from build123d import *

# Parameters (mm, degrees)
SKETCH_1_W          = 80
SKETCH_1_H          = 95
EXTRUDE_1_DEPTH     = 5
CUT_EXTRUDE_2_DEPTH = 10
SKETCH_18_W         = 5
SKETCH_18_H         = 15
CUT_EXTRUDE_4_DEPTH = 10


with BuildPart() as part:
    # 스케치1 → 보스-돌출1 (new body)
    with BuildSketch(Plane(origin=(0, 0, 0), x_dir=(1, 0, 0), z_dir=(0, 1, 0))):
        Rectangle(SKETCH_1_W, SKETCH_1_H)
    extrude(amount=EXTRUDE_1_DEPTH)

    # 스케치9 → 컷-돌출2 (cut)
    with BuildSketch(Plane(origin=(0, 5, 0), x_dir=(1, 0, 0), z_dir=(0, 1, 0))):
        with BuildLine():
            Line((-27, 39.5), (-19, 39.5))
            ThreePointArc((-19, 39.5), (-15.464466094, 38.035533906), (-14, 34.5))
            Line((-14, 34.5), (-14, 21.5))
            ThreePointArc((-14, 21.5), (-15.464466094, 17.964466094), (-19, 16.5))
            Line((-19, 16.5), (-27, 16.5))
            ThreePointArc((-27, 16.5), (-30.535533906, 17.964466094), (-32, 21.5))
            Line((-32, 21.5), (-32, 34.5))
            ThreePointArc((-32, 34.5), (-30.535533906, 38.035533906), (-27, 39.5))
        make_face()
        with BuildLine():
            Line((14, 34.5), (14, 21.5))
            ThreePointArc((14, 21.5), (15.464466094, 17.964466094), (19, 16.5))
            Line((19, 16.5), (27, 16.5))
            ThreePointArc((27, 16.5), (30.535533906, 17.964466094), (32, 21.5))
            Line((32, 21.5), (32, 34.5))
            ThreePointArc((32, 34.5), (30.535533906, 38.035533906), (27, 39.5))
            Line((27, 39.5), (19, 39.5))
            ThreePointArc((19, 39.5), (15.464466094, 38.035533906), (14, 34.5))
        make_face()
        with BuildLine():
            Line((4, 39.5), (-4, 39.5))
            ThreePointArc((-4, 39.5), (-7.535533906, 38.035533906), (-9, 34.5))
            Line((-9, 34.5), (-9, 21.5))
            ThreePointArc((-9, 21.5), (-7.535533906, 17.964466094), (-4, 16.5))
            Line((-4, 16.5), (4, 16.5))
            ThreePointArc((4, 16.5), (7.535533906, 17.964466094), (9, 21.5))
            Line((9, 21.5), (9, 34.5))
            ThreePointArc((9, 34.5), (7.535533906, 38.035533906), (4, 39.5))
        make_face()
        with BuildLine():
            Line((-19, -16.5), (-27, -16.5))
            ThreePointArc((-27, -16.5), (-30.535533906, -17.964466094), (-32, -21.5))
            Line((-32, -21.5), (-32, -34.5))
            ThreePointArc((-32, -34.5), (-30.535533906, -38.035533906), (-27, -39.5))
            Line((-27, -39.5), (-19, -39.5))
            ThreePointArc((-19, -39.5), (-15.464466094, -38.035533906), (-14, -34.5))
            Line((-14, -34.5), (-14, -21.5))
            ThreePointArc((-14, -21.5), (-15.464466094, -17.964466094), (-19, -16.5))
        make_face()
        with BuildLine():
            Line((-19, 11.5), (-27, 11.5))
            ThreePointArc((-27, 11.5), (-30.535533906, 10.035533906), (-32, 6.5))
            Line((-32, 6.5), (-32, -6.5))
            ThreePointArc((-32, -6.5), (-30.535533906, -10.035533906), (-27, -11.5))
            Line((-27, -11.5), (-19, -11.5))
            ThreePointArc((-19, -11.5), (-15.464466094, -10.035533906), (-14, -6.5))
            Line((-14, -6.5), (-14, 6.5))
            ThreePointArc((-14, 6.5), (-15.464466094, 10.035533906), (-19, 11.5))
        make_face()
        with BuildLine():
            Line((-4, 11.5), (4, 11.5))
            ThreePointArc((4, 11.5), (7.535533906, 10.035533906), (9, 6.5))
            Line((9, 6.5), (9, -6.5))
            ThreePointArc((9, -6.5), (7.535533906, -10.035533906), (4, -11.5))
            Line((4, -11.5), (-4, -11.5))
            ThreePointArc((-4, -11.5), (-7.535533906, -10.035533906), (-9, -6.5))
            Line((-9, -6.5), (-9, 6.5))
            ThreePointArc((-9, 6.5), (-7.535533906, 10.035533906), (-4, 11.5))
        make_face()
        with BuildLine():
            Line((19, 11.5), (27, 11.5))
            ThreePointArc((27, 11.5), (30.535533906, 10.035533906), (32, 6.5))
            Line((32, 6.5), (32, -6.5))
            ThreePointArc((32, -6.5), (30.535533906, -10.035533906), (27, -11.5))
            Line((27, -11.5), (19, -11.5))
            ThreePointArc((19, -11.5), (15.464466094, -10.035533906), (14, -6.5))
            Line((14, -6.5), (14, 6.5))
            ThreePointArc((14, 6.5), (15.464466094, 10.035533906), (19, 11.5))
        make_face()
        with BuildLine():
            Line((-4, -16.5), (4, -16.5))
            ThreePointArc((4, -16.5), (7.535533906, -17.964466094), (9, -21.5))
            Line((9, -21.5), (9, -34.5))
            ThreePointArc((9, -34.5), (7.535533906, -38.035533906), (4, -39.5))
            Line((4, -39.5), (-4, -39.5))
            ThreePointArc((-4, -39.5), (-7.535533906, -38.035533906), (-9, -34.5))
            Line((-9, -34.5), (-9, -21.5))
            ThreePointArc((-9, -21.5), (-7.535533906, -17.964466094), (-4, -16.5))
        make_face()
        with BuildLine():
            Line((19, -16.5), (27, -16.5))
            ThreePointArc((27, -16.5), (30.535533906, -17.964466094), (32, -21.5))
            Line((32, -21.5), (32, -34.5))
            ThreePointArc((32, -34.5), (30.535533906, -38.035533906), (27, -39.5))
            Line((27, -39.5), (19, -39.5))
            ThreePointArc((19, -39.5), (15.464466094, -38.035533906), (14, -34.5))
            Line((14, -34.5), (14, -21.5))
            ThreePointArc((14, -21.5), (15.464466094, -17.964466094), (19, -16.5))
        make_face()
    extrude(amount=-CUT_EXTRUDE_2_DEPTH, mode=Mode.SUBTRACT)

    # 스케치18 → 컷-돌출4 (cut)
    with BuildSketch(Plane.XZ):
        with Locations((-37.5, -17.25)):
            Rectangle(SKETCH_18_W, SKETCH_18_H)
        with Locations((-37.5, 17.25)):
            Rectangle(SKETCH_18_W, SKETCH_18_H)
    extrude(amount=-CUT_EXTRUDE_4_DEPTH, mode=Mode.SUBTRACT)


solid = part.part
For this review, take the finished solid that the model builds, in its own axes (mm). A direction names the side the tool comes from. Round coordinates to 2 decimals unless told otherwise and drop trailing zeros. Order: outer loops, then holes, each group sorted by start corner. A loop starts at its lowest first (then second) coordinate and runs counter-clockwise, first axis right, second up. Notation, with made-up numbers: (34, -19) -> (63, -19) arc R18 ccw to (63, -10) -> close; hole circle Ø10 at (-27.5, 81.25). An arc over 180 degrees is marked (long way). Put each result on its own line as item: value.
Q1. Machinability: for faces 1 (the flat face through (-23, 3, 39.5)), 2 (the flat face through (-38, 2, -9.75)), which of the approach directions +Z, -Z, +X, -X, +Y, -Y give a long, thin tool a straight path to every point of the face, cutting with its end or side? Answer none if there is none.
Check result:
face 1: +Y, -Y
face 2: -X, +Y, -Y
Q2. Add section C-C on y = 1.65. State how many separate pieces and enclosed holes the cut face has, plus the area to 3 significant figures.
Check result:
separate pieces: 1
enclosed holes: 9
area: 3,920 mm2
Q3. Add section A-A on z = -4. Write out the cut boundary in (x, y), plus the area to 3 significant figures.
Check result:
outline: (-40, 0) -> (-32, 0) -> (-32, 5) -> (-40, 5) -> close; (-14, 0) -> (-9, 0) -> (-9, 5) -> (-14, 5) -> close; (9, 0) -> (14, 0) -> (14, 5) -> (9, 5) -> close; (32, 0) -> (40, 0) -> (40, 5) -> (32, 5) -> close
area: 130 mm2
Q4. Mouldability with a two-part tool opening along Z and no side actions: class faces 3 (the flat face through (-9, 3, 28)), 4 (the flat face through (40, 2, 1)), 5 (the flat face through (-1, 2, 47.5)) as pulls with the +Z half, pulls with the -Z half, needs draft (parallel to the pull), parting line crosses it, or undercut.
Check result:
face 3: undercut
face 4: needs draft
face 5: pulls with the +Z half
Q5. Add section B-B on x = 7. Write out the cut boundary in (y, z), plus the area to 3 significant figures.
Check result:
outline: (0, -47.5) -> (5, -47.5) -> (5, -38.5) -> (0, -38.5) -> close; (0, -17.5) -> (5, -17.5) -> (5, -10.5) -> (0, -10.5) -> close; (0, 10.5) -> (5, 10.5) -> (5, 17.5) -> (0, 17.5) -> close; (0, 38.5) -> (5, 38.5) -> (5, 47.5) -> (0, 47.5) -> close
area: 160 mm2
Q6. Add section D-D on z = 13. Write out the cut boundary in (x, y), plus the area to 3 significant figures.
Check result:
outline: (-35, 0) -> (40, 0) -> (40, 5) -> (-35, 5) -> close
area: 375 mm2
Q7. Insertion check: pin 1 Ø2.5 at (y, z) = (3, -19) entering from -X; pin 2 Ø3 at (x, z) = (-23, -19) entering from -Y. Each pin has a flat end and moves straight along its axis. Give the tip position at first contact, or say it passes through.
Check result:
pin 1: x = -35
pin 2: through
Q8. For probe 1 along Z at (x, y) = (0.5, 1.45); probe 2 along X at (y, z) = (4.35, -27); probe 3 along X at (y, z) = (2, -19.5), list the stretches that pass through material, from the lowest coordinate up. Write a range as [from, to].
Check result:
probe 1: [-47.5, -39.5], [-16.5, -11.5], [11.5, 16.5], [39.5, 47.5]
probe 2: [-40, -32], [-14, -9], [9, 14], [32, 40]
probe 3: [-35, -31.58], [-14.42, -8.58], [8.58, 14.42], [31.58, 40]
